Could you check a few things on this drawing? It's one solid part, dimensions in mm from its lowest x, y, z. Give positions to 0.01 mm unless a question says otherwise; leave off trailing zeros. Order: outer loops, then holes, each group sorted by start corner. A loop starts at its lowest first (then second) coordinate and runs counter-clockwise, first axis right, second up. Notation, with made-up numbers: (-16, -39.5) -> (5, -39.5) arc R32 cw to (5, -1.5) -> close; hole circle Ø9 at (67.5, -23.75). An arc over 180 degrees is marked (long way). Answer as CSV lines item,"result".
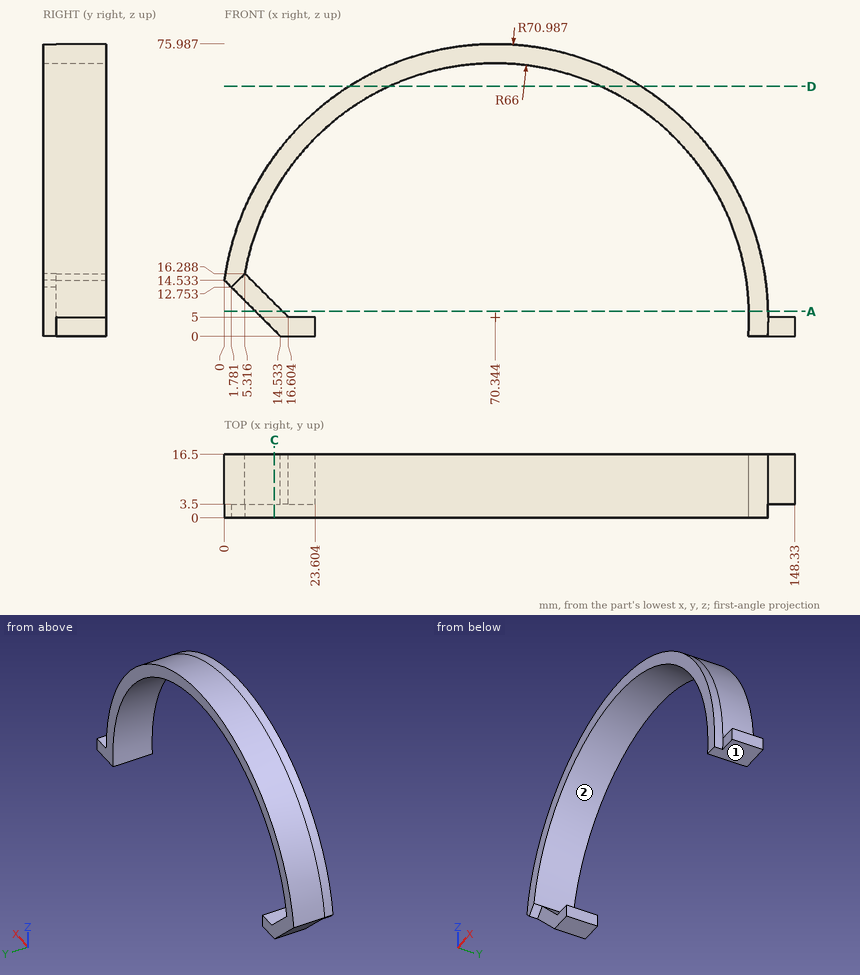
Item 1: Please list where these lines run through material, in increasing order: line 1 along X through (y, z) = (1.25, 35.5) (1 decimal); line 2 along X through (y, z) = (2.75, 50) (1 decimal); line 3 along Z through (x, y) = (56.5, 7).
Numbers:
line 1,"x = 6.2 to 11.8, 128.9 to 134.4"
line 2,"x = 15.4 to 22.1, 118.6 to 125.2"
line 3,"z = 69.53 to 74.62"
Item 2: We'd pull the mould along X, two halves only. Please class the marked faces 1 and 2: released by +X, released by -X, zero draft, split by the parting line, or undercut.
Numbers:
face 1,"zero draft"
face 2,"undercut"
Item 3: For pin 1 (3 mm diameter, centred on y = 5, z = 33.5, fed in from -X); pin 2 (4 mm diameter, centred on y = 13.5, z = 37, fed in from -X); pin 3 (3 mm diameter, centred on x = 101.5, y = 4, fed in from -Z) (1 decimal), each with a flat end and sliding along its axis, tell me the tip position at first contact or that it passes through.
Numbers:
pin 1,"stops at x = 4.69"
pin 2,"stops at x = 6.01"
pin 3,"stops at z = 62.4"
Item 4: Imagine slicing it at D-D, the plane z = 65. Please give me the cut outline in (x, y).
Numbers:
outline,"(32.41, 0) -> (42.85, 0) -> (42.85, 16.5) -> (32.41, 16.5) -> close; (97.84, 0) -> (108.28, 0) -> (108.28, 16.5) -> (97.84, 16.5) -> close"
Item 5: Imagine slicing it at C-C, the plane x = 13. Please give me the cut outline in (y, z) (1 decimal).
Numbers:
outline,"(0, 37.7) -> (16.5, 37.7) -> (16.5, 46.8) -> (0, 46.8) -> close; (3.5, 1.5) -> (16.5, 1.5) -> (16.5, 8.6) -> (3.5, 8.6) -> close"
Item 6: Imagine slicing it at A-A, the plane z = 6.5. Please give me the cut outline in (x, y) (1 decimal).
Numbers:
outline,"(8, 3.5) -> (15.1, 3.5) -> (15.1, 16.5) -> (8, 16.5) -> close; (136.3, 0) -> (141.3, 0) -> (141.3, 16.5) -> (136.3, 16.5) -> close"
